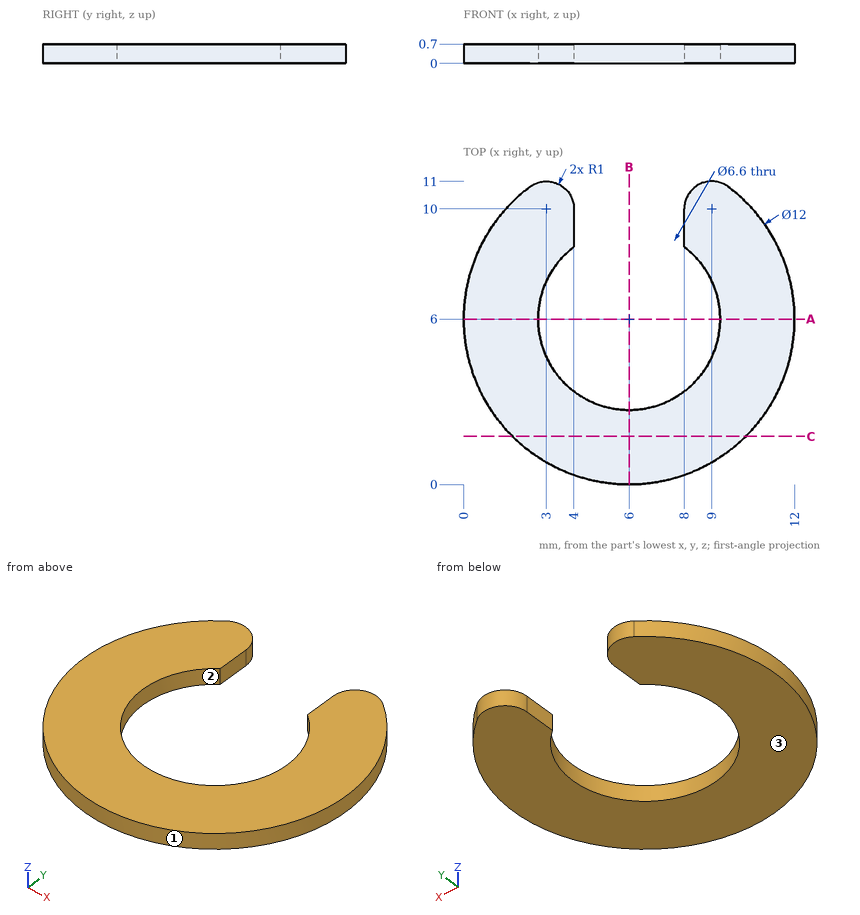
Print and shaded views of the part. All mm, measured from the part's lowest x, y and z. Coordinates: 2 decimals unless noted, no trailing zeros. Loops run counter-clockwise (first coordinate to the right, second up) from the corner with the lowest first, then second, coordinate; pieces in that order, holes last. Notation, with made-up numbers: (26.5, 25.25) - (45.5, 25.25) arc R17 cw to (45.5, 55.25) - close; hole circle Ø10 at (-6, -12). An arc over 180 degrees is marked (long way). Write item = value, one per line. Start each with the question number.
Item 1: Cut at B-B, the plane x = 6. Give the cut face in (y, z), and give its area (3 significant figures).
Item 2: Cut at A-A, the plane y = 6. Give the cut face in (x, z).
Item 3: Cut at C-C, the plane y = 1.75. Give the cut face in (x, z).
Item 4: Mould opens along X. For the marked faces 1, 2 and 3 say: released by +X, released by -X, zero draft, split by the parting line, or undercut.
Item 5: Wall check: L1, parallel to X at y = 6, z = 0.55; L2, parallel to Y at x = 6, z = 0.5; L3, parallel to Y at x = 3, z = 0.65. Give the ranges that are in metal, low to high. Write a range as from..to.
The answers:
q1.outline = (0, 0) - (2.7, 0) - (2.7, 0.7) - (0, 0.7) - close
q1.area = 1.89 mm2
q2.outline = (0, 0) - (2.7, 0) - (2.7, 0.7) - (0, 0.7) - close; (9.3, 0) - (12, 0) - (12, 0.7) - (9.3, 0.7) - close
q3.outline = (1.76, 0) - (10.24, 0) - (10.24, 0.7) - (1.76, 0.7) - close
q4.face_1 = split by the parting line
q4.face_2 = undercut
q4.face_3 = zero draft
q5.L1 = 0..2.7, 9.3..12
q5.L2 = 0..2.7
q5.L3 = 0.8..4.63, 7.37..11
